Build history of the part. All positions in model axes, mm. A direction names the side the tool comes from. Round coordinates to 2 decimals unless told otherwise and drop trailing zeros. Write each loop counter-clockwise with the first axis right and the second up, starting at its lowest first coordinate (ties: lowest second). Pieces come first, ordered by that corner, then holes.
1) Flat gauge pins, fed straight in: pin 1 (11 mm diameter, centred on x = -62, y = 13.5, fed in from +Z); pin 2 (5.5 mm diameter, centred on y = -2.5, z = -2.5, fed in from -X); pin 3 (14.5 mm diameter, centred on y = -1, z = -23.5, fed in from -X). Where does each tip first touch, or does it go through?
2) Saw through at D-D (x = -62). State how many separate pieces and enclosed holes the cut face has, plus the area to 3 significant figures.
3) Wall check: probe 1 along X at (y, z) = (-3.5, -2); probe 2 along X at (y, z) = (1.25, -43.5); probe 3 along Z at (x, y) = (-34, 7.75). Give the ranges that are in metal, low to high.
4) Saw through at A-A (z = -6). Write the cut outline in (x, y).
5) Saw through at B-B (x = 18). Write the cut outline in (y, z), plus the area to 3 significant figures.
6) Which spindle directions (+Z, -Z, +X, -X, +Y, -Y) get a long thin tool onto all of the face, cutting with end or side? Do faces 1 (the flat face through (-62, 9.414, -24)), 2 (the flat face through (55, -2, 1)), 3 (the flat face through (-53, 2, 1)). Say none if no direction does.
7) Saw through at C-C (y = -1.5). Write the cut outline in (x, z), plus the area to 3 significant figures.
8) Pull direction X, two halves, no side cores. Call faces 4 (the flat face through (49, 1, -48)), 5 (the flat face through (57, 5, -1)), 6 (the flat face through (-62, 9.414, 35)): +X half, -X half, draft (parallel to the pull), parting line (faces both ways), or undercut.
Autodesk Inventor part; units mm, degrees
ref_plane "YZ Plane" through (0, 0, 0) normal (1, 0, 0) x (0, 1, 0)
ref_plane "XZ Plane" through (0, 0, 0) normal (0, 1, 0) x (-1, 0, 0)
ref_plane "XY Plane" through (0, 0, 0) normal (0, 0, 1) x (1, 0, 0)
sketch "Esboço3" plane through (0, 0, 0) normal (0, 1, 0) x (-1, 0, 0)
  line L0 (-57, 52) -> (57, 52)
  line L1 (57, 52) -> (57, -52)
  line L2 (57, -52) -> (-57, -52)
  line L3 (-57, -52) -> (-57, 52)
  line L4 (-57, 52) -> (57, -52) construction
  line L5 (57, 52) -> (-57, -52) construction
  line L6 (-53, 48) -> (53, 48)
  line L7 (53, 48) -> (53, -48)
  line L8 (53, -48) -> (-53, -48)
  line L9 (-53, -48) -> (-53, 48)
  line L10 (-53, 48) -> (53, -48) construction
  line L11 (53, 48) -> (-53, -48) construction
  point P0 (0, 0)
  dimension "d9" = 104
  dimension "d10" = 114
  dimension "d11" = 106
  dimension "d12" = 96
extrude "Extrusão2" add sketch "Esboço3" along normal blind 10
sketch "Esboço4" plane through (0, 0, 0) normal (0, -1, 0) x (1, 0, 0)
  line L0 (-53, -48) -> (53, -48)
  line L1 (-53, 48) -> (53, 48)
  line L2 (53, 48) -> (53, -48)
  line L3 (53, -48) -> (-53, -48)
  line L4 (-53, -48) -> (-53, 48)
  line L5 (-53, 48) -> (53, -48) construction
  line L6 (53, 48) -> (-53, -48) construction
  line L7 (-55, 50) -> (55, 50)
  line L8 (55, 50) -> (55, -50)
  line L9 (55, -50) -> (-55, -50)
  line L10 (-55, -50) -> (-55, 50)
  line L11 (-55, 50) -> (55, -50) construction
  line L12 (55, 50) -> (-55, -50) construction
  point P0 (0, 0)
  dimension "d15" = 100
  dimension "d16" = 96
  dimension "d17" = 110
  dimension "d18" = 106
extrude "Extrusão3" add sketch "Esboço4" along normal blind 5
sketch "Esboço5" plane through (0, 10, 0) normal (0, 1, 0) x (1, 0, 0)
  line L0 (53, 48) -> (53, -48)
  line L1 (53, -48) -> (43, -48)
  line L2 (43, -48) -> (43, 48)
  line L3 (43, 48) -> (53, 48)
  line L4 (53, 48) -> (53, -48)
  point P0 (0, 0)
  dimension "d21" = 10
extrude "Extrusão4" add sketch "Esboço5" against normal blind 2
sketch "Esboço6" plane through (0, 8, 0) normal (0, -1, 0) x (1, 0, 0)
  line L0 (43, 48) -> (43, -48)
  line L1 (43, 48) -> (45, 48)
  line L2 (45, 48) -> (45, -48)
  line L3 (45, -48) -> (43, -48)
  line L4 (43, -48) -> (43, 48)
  point P0 (0, 0)
  dimension "d24" = 2
extrude "Extrusão5" add sketch "Esboço6" along normal blind 13
sketch "Esboço7" plane through (0, 10, 0) normal (0, 1, 0) x (1, 0, 0)
  point P0 (0, 0)
sketch "Esboço9" plane through (-57, 0, 52) normal (0, 0, 1) x (1, 0, 0)
  line L0 (114, 0) -> (0, 0)
  line L1 (0, 0) -> (-9.4142, 9.4142)
  line L2 (0, 0) -> (0, 10)
  line L3 (0, 10) -> (-10, 10) construction
  line L4 (0, 10) -> (0, 15.06) construction
  line L5 (0, 15.06) -> (-10, 15.06) construction
  arc A0 (0, 15.06) -> (-10, 15.06) centre (-5, 15.06) ccw
  line L6 (-10, 10.8284) -> (-10, 15.06)
  line L7 (0, 15.06) -> (0, 0)
  circle A1 centre (-5, 15.06) radius 2
  arc A2 (-10, 10.8284) -> (-9.4142, 9.4142) centre (-8, 10.8284) ccw
  point P0 (57, 0)
  dimension "d29" = 45
  dimension "d30" = 5.06
  dimension "d31" = 4
  dimension "d32" = 2
extrude "Extrusão6" add sketch "Esboço9" against normal blind 104
sketch "Esboço10" plane through (-67, 10.8284, 52) normal (-1, 0, 0) x (0, 0, 1)
  line L0 (-52, -10.8284) -> (-67, -10.8284) construction
  line L1 (-102, -10.8284) -> (-2, -10.8284) construction
  line L2 (-67, -10.8284) -> (-37, -10.8284) construction
  line L3 (-37, -10.8284) -> (-37, 9.2316) construction
  line L4 (0, 9.2316) -> (-104, 9.2316) construction
  line L5 (-67, 9.2316) -> (-37, 9.2316) construction
  line L6 (-67, -10.8284) -> (-67, 9.2316) construction
  line L7 (-104, 9.2316) -> (-94.5, 9.2316)
  line L8 (-94.5, 9.2316) -> (-94.5, -10.8284)
  line L9 (-94.5, -10.8284) -> (-104, -10.8284)
  line L10 (-104, -10.8284) -> (-104, 9.2316)
  line L11 (0, 9.2316) -> (-9.5, 9.2316)
  line L12 (-9.5, 9.2316) -> (-9.5, -10.8284)
  line L13 (-9.5, -10.8284) -> (0, -10.8284)
  line L14 (0, -10.8284) -> (0, 9.2316)
  line L15 (-67, 9.2316) -> (-37, 9.2316)
  line L16 (-37, 9.2316) -> (-37, -10.8284)
  line L17 (-37, -10.8284) -> (-67, -10.8284)
  line L18 (-67, -10.8284) -> (-67, 9.2316)
  line L19 (-94.5, 9.2316) -> (-89.5, 9.2316) construction
  line L20 (-9.5, 9.2316) -> (-14.5, 9.2316) construction
  line L21 (-89.5, 9.2316) -> (-83.9, 9.2316)
  line L22 (-83.9, 9.2316) -> (-83.9, -1.4142)
  line L23 (-83.9, -1.4142) -> (-89.5, -1.4142)
  line L24 (-89.5, -1.4142) -> (-89.5, 9.2316)
  line L25 (-14.5, 9.2316) -> (-20.1, 9.2316)
  line L26 (-20.1, 9.2316) -> (-20.1, -1.4142)
  line L27 (-20.1, -1.4142) -> (-14.5, -1.4142)
  line L28 (-14.5, -1.4142) -> (-14.5, 9.2316)
  line L29 (-83.9, 9.2316) -> (-78.9, 9.2316)
  line L30 (-20.1, 9.2316) -> (-25.1, 9.2316)
  line L31 (-78.9, 9.2316) -> (-73.3, 9.2316)
  line L32 (-73.3, 9.2316) -> (-73.3, -1.4142)
  line L33 (-73.3, -1.4142) -> (-78.9, -1.4142)
  line L34 (-78.9, -1.4142) -> (-78.9, 9.2316)
  line L35 (-25.1, 9.2316) -> (-30.7, 9.2316)
  line L36 (-30.7, 9.2316) -> (-30.7, -1.4142)
  line L37 (-30.7, -1.4142) -> (-25.1, -1.4142)
  line L38 (-25.1, -1.4142) -> (-25.1, 9.2316)
  dimension "d35" = 15
  dimension "d36" = 30
  dimension "d37" = 9.5
  dimension "d38" = 9.5
  dimension "d39" = 5
  dimension "d40" = 5
  dimension "d41" = 5.6
  dimension "d42" = 5.6
  dimension "d43" = 5
  dimension "d44" = 5
  dimension "d45" = 5.6
  dimension "d46" = 5.6
extrude "Extrusão7" cut sketch "Esboço10" against normal blind 10
fillet "Arredondamento1" radius 2 4 edges at (57, 5, 52) (57, 5, -52) (-57, 5, -52) (-57, 5, 52)
properties part number "tampa extra"
Evaluation:
1. pin 1: stops at z = 42.5
1. pin 2: stops at x = -57
1. pin 3: stops at x = -63.25
2. separate pieces: 8
2. enclosed holes: 0
2. area: 459 mm2
3. probe 1: x = -55 to -53, 43 to 45, 53 to 55
3. probe 2: x = -57 to -53, 43 to 45, 53 to 57
3. probe 3: z = -52 to -48, 48 to 52
4. outline: (-57, 0) - (-55, 0) - (-55, -5) - (-53, -5) - (-53, 10) - (-57, 10) - close; (43, -5) - (45, -5) - (45, 8) - (53, 8) - (53, -5) - (55, -5) - (55, 0) - (57, 0) - (57, 10) - (43, 10) - close
5. outline: (-5, -50) - (0, -50) - (0, -52) - (10, -52) - (10, -48) - (-5, -48) - close; (-5, 48) - (10, 48) - (10, 52) - (0, 52) - (0, 50) - (-5, 50) - close
5. area: 100 mm2
6. face 1: -X, +Y
6. face 2: +Z, -Z, +X, -Y
6. face 3: +Y, -Y
7. outline: (-55, -50) - (55, -50) - (55, 50) - (-55, 50) - close; hole (-53, -48) - (43, -48) - (43, 48) - (-53, 48) - close; hole (45, -48) - (53, -48) - (53, 48) - (45, 48) - close
7. area: 1,020 mm2
8. face 4: undercut
8. face 5: +X half
8. face 6: draft
